Verification items for this drawing (mm, ordinates from the low corner). Give positions to 0.01 mm unless a question says otherwise; leave off trailing zeros. Loops run counter-clockwise (first coordinate to the right, second up) from the corner with the lowest first, then second, coordinate; pieces in that order, holes last. Notation, with made-up numbers: (78.5, -27.75) -> (129.5, -27.75) arc R16 ccw to (129.5, 2.25) -> close; hole circle Ø5 at (2.5, 76.5). An arc over 180 degrees is marked (long way). Answer as a JSON object with one key per item and string values.
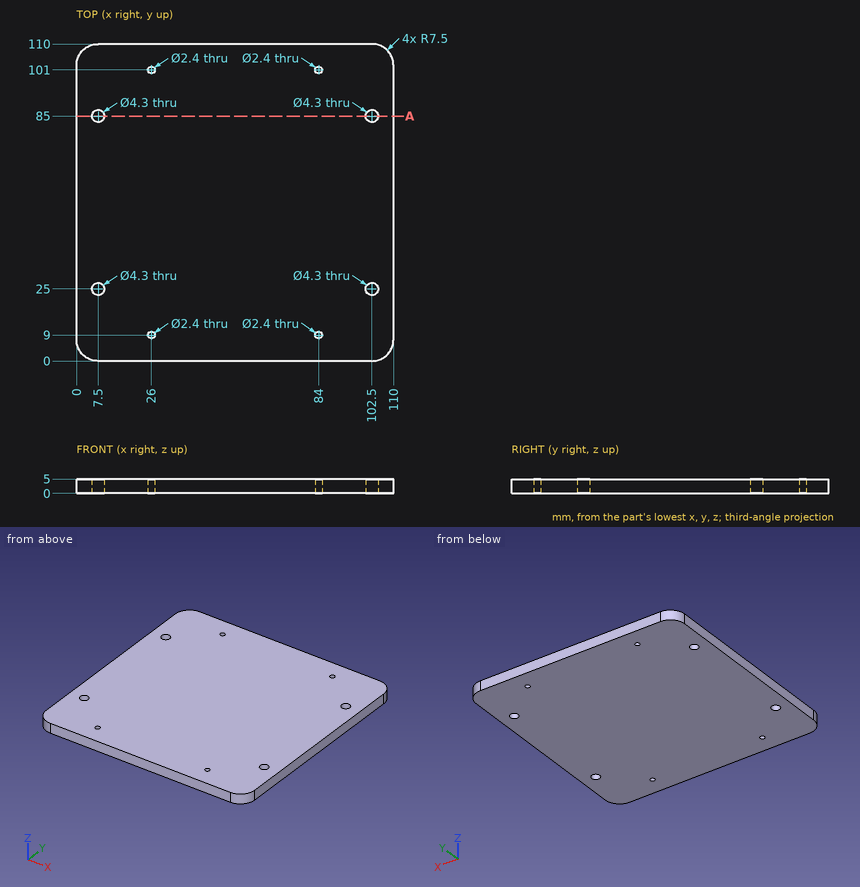
1) Material ranges on line 1 along Y through (x, z) = (7.5, 1.3); line 2 along Y through (x, z) = (26, 4); line 3 along X through (y, z) = (101, 3.6), recorded low to high. Write a range as from..to.
Geometry check:
{"line 1": "y = 0..22.85, 27.15..82.85, 87.15..110", "line 2": "y = 0..7.8, 10.2..99.8, 102.2..110", "line 3": "x = 0..24.8, 27.2..82.8, 85.2..110"}
2) Section check A-A on y = 85. Record the cut outline in (x, z).
Geometry check:
{"outline": "(0, 0) -> (5.35, 0) -> (5.35, 5) -> (0, 5) -> close; (9.65, 0) -> (100.35, 0) -> (100.35, 5) -> (9.65, 5) -> close; (104.65, 0) -> (110, 0) -> (110, 5) -> (104.65, 5) -> close"}
3) Depth check by flat-ended pin: P1, Ø4, axis at x = 102.5, y = 85, coming from the -Z side. Enter the tip coordinate at first touch or a pass-through.
Geometry check:
{"P1": "passes through"}
